```python
from build123d import *

# Parameters (mm, degrees)
SKETCH1_W           = 70.485
SKETCH1_H           = 102.235
BOSS_EXTRUDE1_DEPTH = 28.575
SHELL1_T            = -3.175
SKETCH2_W           = 89.535
SKETCH2_H           = 19.05
CUT_EXTRUDE1_DEPTH  = 3.175
SKETCH3_W           = 67.31
SKETCH3_H           = 19.05
CUT_EXTRUDE2_DEPTH  = 3.175


with BuildPart() as part:
    # Sketch1 → Boss-Extrude1 (new body)
    with BuildSketch(Plane(origin=(0, 0, 0), x_dir=(1, 0, 0), z_dir=(0, 1, 0))):
        with Locations((0.4325, 0.0575)):
            Rectangle(SKETCH1_W, SKETCH1_H)
    extrude(amount=BOSS_EXTRUDE1_DEPTH)

    # Shell1
    shell1_openings = [part.faces().sort_by_distance(p)[0] for p in [
        (0.4325, 28.575, -0.0575),
        (-34.81, 14.2875, -0.0575),
    ]]
    offset(amount=SHELL1_T, openings=shell1_openings, kind=Kind.INTERSECTION)

    # Sketch2 → Cut-Extrude1 (cut)
    with BuildSketch(Plane(origin=(35.675, 0, 0), x_dir=(0, 0, -1), z_dir=(1, 0, 0))):
        with Locations((6.4075, 19.05)):
            Rectangle(SKETCH2_W, SKETCH2_H)
    extrude(amount=-CUT_EXTRUDE1_DEPTH, mode=Mode.SUBTRACT)

    # Sketch3 → Cut-Extrude2 (cut)
    with BuildSketch(Plane(origin=(0, 0, -51.175), x_dir=(-1, 0, 0), z_dir=(0, 0, -1))):
        with Locations((1.155, 19.05)):
            Rectangle(SKETCH3_W, SKETCH3_H)
    extrude(amount=-CUT_EXTRUDE2_DEPTH, mode=Mode.SUBTRACT)


solid = part.part
```
Could you check a few things on this model? Use its own coordinates, in mm. A direction names the side the tool comes from. Coordinates: 2 decimals unless noted, no trailing zeros. Write each loop counter-clockwise with the first axis right and the second up, starting at its lowest first coordinate (ties: lowest second). Pieces come first, ordered by that corner, then holes. Notation, with made-up numbers: (-24.75, 59.5) -> (29.25, 59.5) arc R21 cw to (29.25, 78.5) -> close; hole circle Ø3 at (8, 33.25). An arc over 180 degrees is marked (long way). One line per question, with ' | ' between items. Start each with the question number.
1. Please list where these lines run through material, in increasing order: line 1 along Z through (x, y) = (9, 6.75) (3 decimals); line 2 along Z through (x, y) = (-29, 21) (3 decimals); line 3 along Y through (x, z) = (-5, 32) (3 decimals).
2. Will these pins go through, and if not, where does the flat tip stop? P1, Ø21, axis at x = -11, z = 8, coming from the +Y side (3 decimals); P2, Ø2, axis at y = 22, z = 37.5, coming from the +X side (3 decimals); P3, Ø5, axis at y = 25, z = 34.5, coming from the +X side; P4, Ø4, axis at x = -5, y = 13, coming from the -Z side (3 decimals).
3. If we section it at C-C (z = 30): Please give me the cut outline in (x, y) (3 decimals), and give its area (3 significant figures).
4. If we section it at A-A (x = -17): Please give me the cut outline in (y, z) (3 decimals), and give its area (3 significant figures).
5. If we section it at D-D (y = 5): Please give me the cut outline in (x, z) (3 decimals), and give its area (3 significant figures).
6. For faces 4 (the face through (32.5, 9, 11)), 5 (the face through (-34.81, 2, 8)), which set-ups out of +Z, -Z, +X, -X, +Y, -Y let a thin tool reach every point of the face, with its end or its side?
7. Thinking about a two-plate mould opening in Z: for faces 1 (the face through (35, 9.525, -27)), 2 (the face through (-2, 6, -48)), 3 (the face through (34, 19, 38.36)), which applies, pulls with the +Z half, pulls with the -Z half, needs draft (parallel to the pull), parting line crosses it, or undercut?
8. If we section it at B-B (y = 11): Please give me the cut outline in (x, z) (3 decimals), and give its area (3 significant figures).
Return value:
1) line 1: z = -51.175 to -48, 47.885 to 51.06 | line 2: z = 47.885 to 51.06 | line 3: y = 0 to 3.175
2) P1: stops at y = 3.175 | P2: stops at x = 35.675 | P3: passes through | P4: stops at z = 47.885
3) outline: (-34.81, 0) -> (35.675, 0) -> (35.675, 9.525) -> (32.5, 9.525) -> (32.5, 3.175) -> (-34.81, 3.175) -> close | area: 244 mm²
4) outline: (0, -51.175) -> (9.525, -51.175) -> (9.525, -48) -> (3.175, -48) -> (3.175, 47.885) -> (28.575, 47.885) -> (28.575, 51.06) -> (0, 51.06) -> close | area: 425 mm²
5) outline: (-34.81, -51.175) -> (35.675, -51.175) -> (35.675, 51.06) -> (-34.81, 51.06) -> (-34.81, 47.885) -> (32.5, 47.885) -> (32.5, -48) -> (-34.81, -48) -> close | area: 752 mm²
6) face 4: -X, +Y | face 5: +Z, -Z, -X, +Y, -Y
7) face 1: needs draft | face 2: undercut | face 3: pulls with the -Z half
8) outline: (-34.81, 47.885) -> (32.5, 47.885) -> (32.5, 38.36) -> (35.675, 38.36) -> (35.675, 51.06) -> (-34.81, 51.06) -> close | area: 254 mm²
